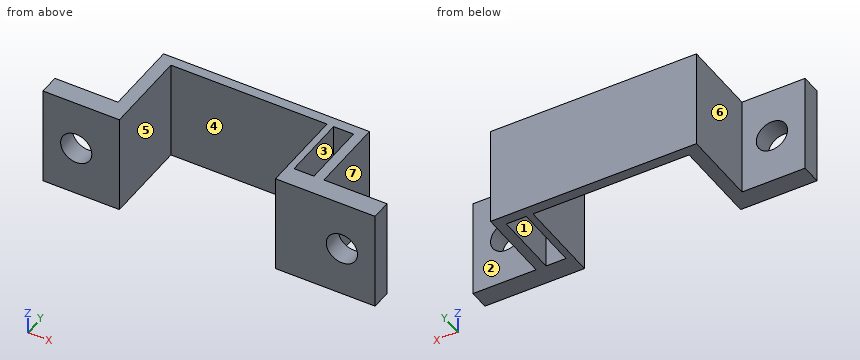
```python
from build123d import *

# Parameters (mm, degrees)
SKETCH001_AS_DRAWN_R                 = 2.35
EXTRUDE001_DEPTH                     = 5
EXTRUDE001_ONTO_SKETCH001_ROLL_ANGLE = 90
SKETCH_W                             = 3
SKETCH_H                             = 10
EXTRUDE_DEPTH                        = 15


with BuildPart() as extrude001:
    # Sketch001 as drawn → Extrude001 (new)
    with BuildSketch(Plane.XY):
        with Locations((-20, 7.5)):
            Circle(SKETCH001_AS_DRAWN_R)
        with Locations((20, 7.5)):
            Circle(SKETCH001_AS_DRAWN_R)
    extrude(amount=-EXTRUDE001_DEPTH)


with BuildPart() as extrude001_1:
    # Extrude001 onto Sketch001 roll: moved
    add(extrude001.part.rotate(Axis((0, 0, 0), (1, 0, 0)), EXTRUDE001_ONTO_SKETCH001_ROLL_ANGLE))


with BuildPart() as extrude001_2:
    # Extrude001 onto Sketch001 placement: moved
    add(extrude001_1.part)


with BuildPart() as cut:
    # Sketch → Extrude (new body)
    with BuildSketch(Plane.XY):
        Polygon((-25, 0), (-13.5, 0), (-13.5, 13), (10, 13), (10, 0), (25, 0), (25, 3), (15.5, 3), (15.5, 14.5), (-15.5, 14.5), (-15.5, 3), (-25, 3), align=None)
        with Locations((12.5, 8)):
            Rectangle(SKETCH_W, SKETCH_H, mode=Mode.SUBTRACT)
    extrude(amount=EXTRUDE_DEPTH)

    # Cut: cut Extrude001
    add(extrude001_2.part, mode=Mode.SUBTRACT)


solid = cut.part
```
CAD build for the part. Positions are in the model's coordinates, mm. Face numbers are marked on the shaded views. A direction names the side the tool comes from. Round coordinates to 2 decimals unless told otherwise and drop trailing zeros. Write each loop counter-clockwise with the first axis right and the second up, starting at its lowest first coordinate (ties: lowest second). Pieces come first, ordered by that corner, then holes. Notation, with made-up numbers: (37, 42) - (51, 42) arc R33 cw to (51, 80) - close; hole circle Ø9 at (63.5, 46). An arc over 180 degrees is marked (long way). Return JSON: item names as keys, results as strings. Group by question number.
Item 1: Probe probe 1 along X at (y, z) = (10.5, 7.5); probe 2 along X at (y, z) = (2.5, 12.5); probe 3 along Z at (x, y) = (20, 2.35). List the from-to ranges inside material, lowest first.
Item 2: Band-saw the part on C-C on x = 12. List the corners of the cut face in (y, z).
Item 3: Mould opens along Y. For the marked faces 1, 2, 3 and 4 say: +Y half, -Y half, draft (parallel to the pull), parting line (faces both ways), or undercut.
Item 4: 3-axis set-ups, long thin cutter, end or side, ignore diameter. For the marked faces 5, 6 and 7: which of +Z, -Z, +X, -X, +Y, -Y reach the whole face in a straight line?
Item 5: Flat gauge pins, fed straight in: pin 1 Ø8 at (x, z) = (0, 8) entering from -Y; pin 2 Ø3 at (x, z) = (20, 7.5) entering from -Y; pin 3 Ø4 at (y, z) = (7.5, 11) entering from +X; pin 4 Ø6 at (y, z) = (8, 8.5) entering from -X. Where does each tip first touch, or does it go through?
Item 6: Band-saw the part on A-A on z = 7.5. List the corners of the cut face in (x, y).
Item 7: Band-saw the part on B-B on y = 1. List the corners of the cut face in (x, z).
Item 8: Band-saw the part on D-D on z = 12.25. List the corners of the cut face in (x, y).
Resolved:
{
 "1": {"probe 1": "x = -15.5 to -13.5, 10 to 11, 14 to 15.5", "probe 2": "x = -25 to -13.5, 10 to 25", "probe 3": "z = 0 to 5.15, 9.85 to 15"},
 "2": {"outline": "(0, 0) - (3, 0) - (3, 15) - (0, 15) - close; (13, 0) - (14.5, 0) - (14.5, 15) - (13, 15) - close"},
 "3": {"face 1": "undercut", "face 2": "+Y half", "face 3": "undercut", "face 4": "-Y half"},
 "4": {"face 5": "+Z, -Z, -Y", "face 6": "+Z, -Z, -X, +Y", "face 7": "+Z, -Z, +X, +Y"},
 "5": {"pin 1": "stops at y = 13", "pin 2": "passes through", "pin 3": "stops at x = 15.5", "pin 4": "stops at x = -15.5"},
 "6": {"outline": "(-25, 0) - (-22.35, 0) - (-22.35, 3) - (-25, 3) - close; (-17.65, 0) - (-13.5, 0) - (-13.5, 13) - (10, 13) - (10, 0) - (17.65, 0) - (17.65, 3) - (15.5, 3) - (15.5, 14.5) - (-15.5, 14.5) - (-15.5, 3) - (-17.65, 3) - close; (22.35, 0) - (25, 0) - (25, 3) - (22.35, 3) - close; hole (11, 3) - (14, 3) - (14, 13) - (11, 13) - close"},
 "7": {"outline": "(-25, 0) - (-13.5, 0) - (-13.5, 15) - (-25, 15) - close; (10, 0) - (25, 0) - (25, 15) - (10, 15) - close; hole circle Ø4.7 at (-20, 7.5); hole circle Ø4.7 at (20, 7.5)"},
 "8": {"outline": "(-25, 0) - (-13.5, 0) - (-13.5, 13) - (10, 13) - (10, 0) - (25, 0) - (25, 3) - (15.5, 3) - (15.5, 14.5) - (-15.5, 14.5) - (-15.5, 3) - (-25, 3) - close; hole (11, 3) - (14, 3) - (14, 13) - (11, 13) - close"}
}
